from build123d import *

# Parameters (mm, degrees)
F0_R     = 12.9
F1_DEPTH = 9
F2_R     = 9
F3_DEPTH = 6
F4_R     = 2.5
F5_DEPTH = 25
F6_W     = 1.571994
F6_H     = 7
F8_R     = 1.75
F9_DEPTH = 25


with BuildPart() as f1:
    # F0 (on Top) → F1 (new body)
    with BuildSketch(Plane.XY):
        Circle(F0_R)
    extrude(amount=F1_DEPTH)

    # F2 (on face) → F3 (join)
    with BuildSketch(Plane(origin=(0, 0, 0), x_dir=(1, 0, 0), z_dir=(0, 0, -1))):
        Circle(F2_R)
    extrude(amount=F3_DEPTH)

    # F4 (on face) → F5 (cut)
    with BuildSketch(Plane(origin=(0, 0, -6), x_dir=(1, 0, 0), z_dir=(0, 0, -1))):
        Circle(F4_R)
    extrude(amount=-F5_DEPTH, mode=Mode.SUBTRACT)

    # F6 (on Front) → F7 (revolve, cut)
    with BuildSketch(Plane.XZ):
        with Locations((-13.285997, 4.5)):
            Rectangle(F6_W, F6_H)
    revolve(axis=Axis((0, 0, 9), (0, 0, -1)), mode=Mode.SUBTRACT)

    # F8 (on Front) → F9 (cut)
    with BuildSketch(Plane.XZ):
        with Locations((0, -3)):
            Circle(F8_R)
    extrude(amount=-F9_DEPTH, mode=Mode.SUBTRACT)


solid = f1.part
Design review of the part built by this model. Coordinates are the model's own, in mm. A direction names the side the tool comes from. Give positions to 0.01 mm unless a question says otherwise; leave off trailing zeros. Loops run counter-clockwise (first coordinate to the right, second up) from the corner with the lowest first, then second, coordinate; pieces in that order, holes last. Notation, with made-up numbers: M -6.75,45.5 L 20.25,45.5 A9 cw 20.25,49.5 Z; hole C 46,27 d5. An arc over 180 degrees is marked long. Answer as a JSON object with one key per item and string values.
Item 1: We need section B-B (y = 0). State the section outline as (x, z) points, and give its area (3 significant figures).
Output values:
{"outline": "M -12.9,0 L -9,0 L -9,-6 L -2.5,-6 L -2.5,9 L -12.9,9 L -12.9,8 L -12.5,8 L -12.5,1 L -12.9,1 Z; M 2.5,-6 L 9,-6 L 9,0 L 12.9,0 L 12.9,1 L 12.5,1 L 12.5,8 L 12.9,8 L 12.9,9 L 2.5,9 Z", "area": "260 mm2"}
Item 2: Machinability: for faces 1 (the face through (-11.923, 3.755, 4.549)), 2 (the face through (-1.172, -8.923, -2.958)), 3 (the face through (0, -3, 9)), which of the approach directions +Z, -Z, +X, -X, +Y, -Y give a long, thin tool a straight path to every point of the face, cutting with its end or side? Answer none if there is none.
Output values:
{"face 1": "none", "face 2": "-Z", "face 3": "+Z, +X, -X, +Y, -Y"}
Item 3: We need section C-C (y = 4.5). State the section outline as (x, z) points.
Output values:
{"outline": "M -12.09,0 L -7.79,0 L -7.79,-6 L 7.79,-6 L 7.79,0 L 12.09,0 L 12.09,1 L 11.66,1 L 11.66,8 L 12.09,8 L 12.09,9 L -12.09,9 L -12.09,8 L -11.66,8 L -11.66,1 L -12.09,1 Z; hole C 0,-3 d3.5"}
Item 4: Mouldability with a two-part tool opening along Y and no side actions: class faces 4 (the face through (-0.33, -2.48, 1.39)), 5 (the face through (-2.796, -12.593, 8.493)), 6 (the face through (-0.38, 5.34, -4.71)) as pulls with the +Y half, pulls with the -Y half, needs draft (parallel to the pull), parting line crosses it, or undercut.
Output values:
{"face 4": "undercut", "face 5": "parting line crosses it", "face 6": "needs draft"}
Item 5: Wall thickness on line 1 along Y through (x, z) = (0, 2.5); line 2 along Z through (x, y) = (11.75, 3.5); line 3 along Y through (x, z) = (0, 0.25): over which ranges is each line inside the solid? List them lowest first.
Output values:
{"line 1": "y = -12.5 to -2.5, 2.5 to 12.5", "line 2": "z = 0 to 9", "line 3": "y = -12.9 to -2.5, 2.5 to 12.9"}
Item 6: For P1, Ø1.5, axis at x = 1.5, z = 1.5, coming from the +Y side; P2, Ø1.5, axis at y = -7, z = 2.5, coming from the -X side; P3, Ø3, axis at x = 0, z = -3, coming from the -Y side, all flat-tipped, find the tip position at first contact; note any pin that passes through.
Output values:
{"P1": "stops at y = 12.87", "P2": "stops at x = -10.83", "P3": "stops at y = -9"}
Item 7: We need section A-A (x = 0). State the section outline as (y, z) points, and give its area (3 significant figures).
Output values:
{"outline": "M -12.9,0 L -9,0 L -9,-6 L -2.5,-6 L -2.5,9 L -12.9,9 L -12.9,8 L -12.5,8 L -12.5,1 L -12.9,1 Z; M 2.5,-6 L 9,-6 L 9,-4.75 L 2.5,-4.75 Z; M 2.5,-1.25 L 9,-1.25 L 9,0 L 12.9,0 L 12.9,1 L 12.5,1 L 12.5,8 L 12.9,8 L 12.9,9 L 2.5,9 Z", "area": "237 mm2"}
Item 8: We need section D-D (y = -10.5). State the section outline as (x, z) points, and give its area (3 significant figures).
Output values:
{"outline": "M -7.49,0 L 7.49,0 L 7.49,1 L 6.78,1 L 6.78,8 L 7.49,8 L 7.49,9 L -7.49,9 L -7.49,8 L -6.78,8 L -6.78,1 L -7.49,1 Z", "area": "125 mm2"}
